from build123d import *

# Parameters (mm, degrees)
ESQUISSE1_W              = 20
ESQUISSE1_H              = 41
BOSS_EXTRU_1_DEPTH       = 37.7
CONG_1_R                 = 1
BOSS_EXTRU_2_DEPTH       = 6.5
BOSS_EXTRU_2_DEPTH_BACK  = 47.5
ESQUISSE2_W              = 19
ESQUISSE2_H              = 2.5
ESQUISSE3_R              = 6.4
BOSS_EXTRU_3_DEPTH       = 1
ESQUISSE4_R              = 2.75
BOSS_EXTRU_4_DEPTH       = 4
ENL_V_MAT_EXTRU_1_DEPTH  = 4
ESQUISSE6_W              = 6.5
ESQUISSE6_H              = 4.5
BOSS_EXTRU_6_DEPTH       = 2.8
BOSS_EXTRU_6_TAPER       = 10
BOSS_EXTRU_12_DEPTH      = 2.2
BOSS_EXTRU_13_DEPTH      = 0.5
BOSS_EXTRU_13_DEPTH_BACK = 0.5
ESQUISSE8_W              = 34.833277075
ESQUISSE8_H              = 46.278938305
ENL_V_MAT_EXTRU_2_DEPTH  = 2
CONG_2_R                 = 1
ESQUISSE9_R              = 5.5
BOSS_EXTRU_14_DEPTH      = 0.25


with BuildPart() as part:
    # Esquisse1 → Boss.-Extru.1 (new body)
    with BuildSketch(Plane.XY):
        with Locations((10, 20.5)):
            Rectangle(ESQUISSE1_W, ESQUISSE1_H)
    extrude(amount=BOSS_EXTRU_1_DEPTH)

    # Congé1
    cong_1_edges = [part.edges().sort_by_distance(p)[0] for p in [
        (0, 41, 18.85),
        (20, 41, 18.85),
        (20, 0, 18.85),
        (0, 0, 18.85),
    ]]
    fillet(cong_1_edges, radius=CONG_1_R)

    # Esquisse2 → Boss.-Extru.2 (add, two sides: drawn at the far end of the back side and taken through both)
    with BuildSketch(Plane.XZ.offset(-BOSS_EXTRU_2_DEPTH_BACK)):
        with Locations((10, 28.25)):
            Rectangle(ESQUISSE2_W, ESQUISSE2_H)
    extrude(amount=BOSS_EXTRU_2_DEPTH + BOSS_EXTRU_2_DEPTH_BACK)

    # Esquisse3 → Boss.-Extru.3 (add)
    with BuildSketch(Plane.XY.offset(37.7)):
        with Locations(Location((10, 31, 0), (0, 0, 180))):
            Circle(ESQUISSE3_R)
    extrude(amount=BOSS_EXTRU_3_DEPTH)

    # Esquisse4 → Boss.-Extru.4 (add)
    with BuildSketch(Plane.XY.offset(38.7)):
        with Locations((10, 31)):
            Circle(ESQUISSE4_R)
    extrude(amount=BOSS_EXTRU_4_DEPTH)

    # Esquisse5 → Enlèv. mat.-Extru.1 (cut)
    with BuildSketch(Plane.XY.offset(29.5)):
        with BuildLine():
            ThreePointArc((16, 46.232050808), (15, 42.5), (14, 46.232050808))
            Line((14, 46.232050808), (14, 48.5))
            Line((14, 48.5), (16, 48.5))
            Line((16, 48.5), (16, 46.232050808))
        make_face()
        with BuildLine():
            Line((4, 48.5), (4, 46.232050808))
            ThreePointArc((4, 46.232050808), (5, 42.5), (6, 46.232050808))
            Line((6, 46.232050808), (6, 48.5))
            Line((6, 48.5), (4, 48.5))
        make_face()
        with BuildLine():
            Line((4, -6.5), (6, -6.5))
            Line((6, -6.5), (6, -5.232050808))
            ThreePointArc((6, -5.232050808), (5, -1.5), (4, -5.232050808))
            Line((4, -5.232050808), (4, -6.5))
        make_face()
        with BuildLine():
            Line((14, -6.5), (16, -6.5))
            Line((16, -6.5), (16, -5.232050808))
            ThreePointArc((16, -5.232050808), (15, -1.5), (14, -5.232050808))
            Line((14, -5.232050808), (14, -6.5))
        make_face()
    extrude(amount=-ENL_V_MAT_EXTRU_1_DEPTH, mode=Mode.SUBTRACT)

    # Esquisse6 → Boss.-Extru.6 (add)
    with BuildSketch(Plane(origin=(0, 41, 0), x_dir=(1, 0, 0), z_dir=(0, 1, 0))):
        with Locations((10, -4.75)):
            Rectangle(ESQUISSE6_W, ESQUISSE6_H)
    extrude(amount=BOSS_EXTRU_6_DEPTH, taper=BOSS_EXTRU_6_TAPER)

    # Esquisse7 → Boss.-Extru.12 (add)
    with BuildSketch(Plane(origin=(0, 43.8, 0), x_dir=(1, 0, 0), z_dir=(0, 1, 0))):
        with BuildLine():
            Line((10.751668523, -4.8), (10.748331477, -4.8))
            ThreePointArc((10.748331477, -4.8), (10, -5.5), (9.251668523, -4.8))
            Line((9.251668523, -4.8), (9.248331477, -4.8))
            ThreePointArc((9.248331477, -4.8), (7.75, -4.75), (9.248331477, -4.7))
            Line((9.248331477, -4.7), (9.251668523, -4.7))
            ThreePointArc((9.251668523, -4.7), (10, -4), (10.748331477, -4.7))
            Line((10.748331477, -4.7), (10.751668523, -4.7))
            ThreePointArc((10.751668523, -4.7), (12.25, -4.75), (10.751668523, -4.8))
        make_face()
    extrude(amount=BOSS_EXTRU_12_DEPTH)

    # Esquisse3D1 → Boss.-Extru.13 (add, two sides: drawn at the far end of the back side and taken through both)
    with BuildSketch(Plane(origin=(10, -6.5, 29.5), x_dir=(0, 1, 0), z_dir=(1, 0, 0)).offset(-BOSS_EXTRU_13_DEPTH_BACK)):
        Polygon((0, 0), (6.5, 0), (6.5, 1.5), align=None)
        Polygon((54, 0), (47.5, 0), (47.5, 1.5), align=None)
    extrude(amount=BOSS_EXTRU_13_DEPTH + BOSS_EXTRU_13_DEPTH_BACK)

    # Esquisse8 → Enlèv. mat.-Extru.2 (cut)
    with BuildSketch(Plane.XY.offset(37.7)):
        with Locations((11.272378628, 21.882709323)):
            Rectangle(ESQUISSE8_W, ESQUISSE8_H)
        with BuildLine():
            Line((1, 26.641101056), (1, 7.5))
            Line((1, 7.5), (5, 7.5))
            ThreePointArc((5, 7.5), (10, 3.896834669), (15, 7.5))
            Line((15, 7.5), (19, 7.5))
            Line((19, 7.5), (19, 26.641101056))
            ThreePointArc((19, 26.641101056), (10, 41), (1, 26.641101056))
        make_face(mode=Mode.SUBTRACT)
    extrude(amount=-ENL_V_MAT_EXTRU_2_DEPTH, mode=Mode.SUBTRACT)

    # Congé2
    cong_2_edges = [part.edges().sort_by_distance(p)[0] for p in [
        (0.5, 47.5, 28.25),
        (19.5, 47.5, 28.25),
        (0.5, -6.5, 28.25),
        (19.5, -6.5, 28.25),
    ]]
    fillet(cong_2_edges, radius=CONG_2_R)

    # Esquisse9 → Boss.-Extru.14 (add)
    with BuildSketch(Plane.XY.offset(38.7)):
        with Locations((10, 31)):
            Circle(ESQUISSE9_R)
    extrude(amount=BOSS_EXTRU_14_DEPTH)


solid = part.part
Geometry: final body of the model. Coordinates: model frame, mm. A direction names the side the tool comes from. Round coordinates to 2 decimals unless told otherwise and drop trailing zeros. Loops run counter-clockwise (first coordinate to the right, second up) from the corner with the lowest first, then second, coordinate; pieces in that order, holes last. Notation, with made-up numbers: M 40.5,64 L 45.5,64 A19 cw 45.5,74 Z; hole C -19.5,32 d6. An arc over 180 degrees is marked long. Put each result on its own line as item: value. Start each with the question number.
(1) Material intervals for line 1 along X through (y, z) = (-3.5, 28); line 2 along X through (y, z) = (-3, 28); line 3 along Z through (x, y) = (9, 16), sorted ascending. Write a range as [from, to].
(2) Set-up query: faces 1 (the face through (9.5, 43, 30)), 2 (the face through (11, 34, 38.95)), 3 (the face through (4, 47, 28)). Return all of +Z, -Z, +X, -X, +Y, -Y with unobstructed straight access to the full face (end or side cutting, diameter ignored); none if empty.
(3) Contact query for flat-ended pins moving along their axis: pin 1 Ø3 at (x, y) = (3.5, 30) entering from +Z; pin 2 Ø10 at (x, z) = (6.5, 38.5) entering from -Y; pin 3 Ø5.5 at (x, y) = (12.5, 44) entering from -Z; pin 4 Ø10 at (x, y) = (9.5, 30.5) entering from -Z. Output: stop coordinate, or through.
(4) Section query B-B (y = 14). Return loops of the section in (x, z), then the cut area to 3 significant figures.
(5) Draft query along Z for faces 4 (the face through (10, 46, 5)), 5 (the face through (10, 44, 27)), 6 (the face through (10, 21, 0)), 7 (the face through (3, 43, 29.5)). Return one class per face: +Z half, -Z half, draft (parallel to the pull), parting line (faces both ways), or undercut.
(6) Section query A-A (z = 20). Return loops of the section in (x, y), then the cut area to 3 significant figures.
Findings below:
1. line 1: x = [0.5, 3], [7, 13], [17, 19.5]
1. line 2: x = [0.5, 3.06], [6.94, 13.06], [16.94, 19.5]
1. line 3: z = [0, 37.7]
2. face 1: +Z, -X, +Y
2. face 2: +Z
2. face 3: +Z, -Z, +Y
3. pin 1: stops at z = 38.95
3. pin 2: stops at y = 0
3. pin 3: stops at z = 2.54
3. pin 4: stops at z = 0
4. outline: M 0,0 L 20,0 L 20,35.7 L 19,35.7 L 19,37.7 L 1,37.7 L 1,35.7 L 0,35.7 Z
4. area: 750 mm2
5. face 4: draft
5. face 5: undercut
5. face 6: -Z half
5. face 7: +Z half
6. outline: M 0,1 A1 ccw 1,0 L 19,0 A1 ccw 20,1 L 20,40 A1 ccw 19,41 L 1,41 A1 ccw 0,40 Z
6. area: 819 mm2
